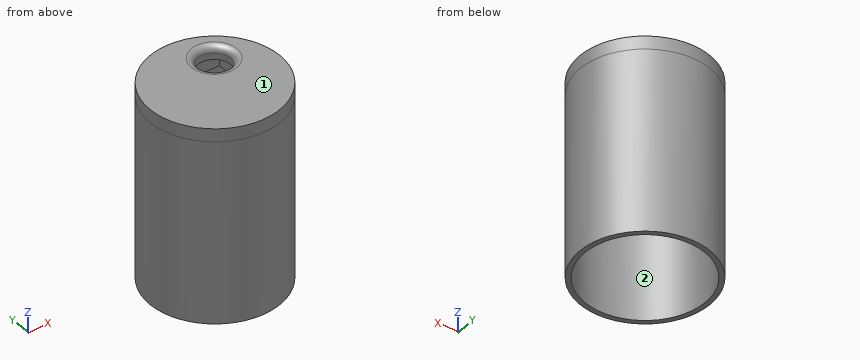
```python
from build123d import *

# Parameters (mm, degrees)
SKETCH_R      = 10
SKETCH_R_2    = 9.25
PAD_DEPTH     = 28
SKETCH001_R   = 10
SKETCH001_W   = 10.7
SKETCH001_H   = 13.5
PAD001_DEPTH  = 2
SKETCH005_R   = 10
SKETCH005_R_2 = 2.5
PAD004_DEPTH  = 2
FILLET_R      = 1


with BuildPart() as part:
    # Sketch (on XY_Plane of Origin) → Pad (new body)
    with BuildSketch(Plane.XY):
        with Locations((12, 10.7)):
            Circle(SKETCH_R)
        with Locations((12, 10.7)):
            Circle(SKETCH_R_2, mode=Mode.SUBTRACT)
    extrude(amount=-PAD_DEPTH)

    # Sketch001 (on Face3 of Pad) → Pad001 (join)
    with BuildSketch(Plane.XY):
        with Locations((12, 10.7)):
            Circle(SKETCH001_R)
        with Locations((12.5, 11.05)):
            Rectangle(SKETCH001_W, SKETCH001_H, mode=Mode.SUBTRACT)
    extrude(amount=-PAD001_DEPTH)

    # Sketch005 (on Face8 of Pad001) → Pad004 (join)
    with BuildSketch(Plane.XY):
        with Locations((12, 10.7)):
            Circle(SKETCH005_R)
        with Locations((15, 15)):
            Circle(SKETCH005_R_2, mode=Mode.SUBTRACT)
    extrude(amount=PAD004_DEPTH)

    # Fillet
    fillet_edges = [part.edges().sort_by_distance(p)[0] for p in [
        (12.5, 15, 2),
    ]]
    fillet(fillet_edges, radius=FILLET_R)


solid = part.part
```
Source: CAD feature listing. Evaluate the final solid. Frame: model axes, mm. Face numbers are marked on the shaded views. Round coordinates to 2 decimals unless told otherwise and drop trailing zeros. Order: outer loops, then holes, each group sorted by start corner. A loop starts at its lowest first (then second) coordinate and runs counter-clockwise, first axis right, second up. Notation, with made-up numbers: (14.5, -3) -> (65.5, -3) arc R19 cw to (65.5, 26) -> close; hole circle Ø8 at (4, -19.75). An arc over 180 degrees is marked (long way). Use CSV: the item, a comma, the result in double quotes.
(1) First-contact query: pin 1 Ø0.6 at (x, z) = (14, -1) entering from -Y; pin 2 Ø5.5 at (x, y) = (10, 8) entering from -Z; pin 3 Ø2 at (x, z) = (14, -1) entering from +Y. Flat tips, straight axial feed; report the tip coordinate or a pass-through.
Report:
pin 1,"y = 0.85"
pin 2,"z = 0"
pin 3,"y = 20.65"
(2) Pull-direction query (Y, two-part tool) for the marked faces 1 and 2; classes: +Y half, -Y half, draft (parallel to the pull), parting line (faces both ways), or undercut.
Report:
face 1,"draft"
face 2,"undercut"
(3) Ray query, L1, parallel to X at y = 10.5, z = -9; L2, parallel to Y at x = 12, z = -16; L3, parallel to Z at x = 18.5, y = 4.5. Return the intervals inside material, ascending.
Report:
L1,"2 to 2.75, 21.25 to 22"
L2,"0.7 to 1.45, 19.95 to 20.7"
L3,"-2 to 2"
(4) Section B-B on y = 15. Return the cut outline in (x, z), and give its area (3 significant figures).
Report:
outline,"(2.97, -28) -> (3.81, -28) -> (3.81, -2) -> (7.15, -2) -> (7.15, 0) -> (12.5, 0) -> (12.5, 1) arc R1 ccw to (11.5, 2) -> (2.97, 2) -> close; (17.5, 0) -> (17.85, 0) -> (17.85, -2) -> (20.19, -2) -> (20.19, -28) -> (21.03, -28) -> (21.03, 2) -> (18.5, 2) arc R1 ccw to (17.5, 1) -> close"
area,"84.0 mm^2"
(5) Section D-D on y = 10.7. Return the cut outline in (x, z), and give its area (3 significant figures).
Report:
outline,"(2, -28) -> (2.75, -28) -> (2.75, -2) -> (7.15, -2) -> (7.15, 0) -> (17.85, 0) -> (17.85, -2) -> (21.25, -2) -> (21.25, -28) -> (22, -28) -> (22, 2) -> (2, 2) -> close"
area,"97.6 mm^2"
(6) Section C-C on z = -9.5. Return the cut outline in (x, y), and give its area (3 significant figures).
Report:
outline,"circle Ø20 at (12, 10.7); hole circle Ø18.5 at (12, 10.7)"
area,"45.4 mm^2"
(7) Section A-A on x = 15. Return the cut outline in (y, z).
Report:
outline,"(1.16, -28) -> (1.95, -28) -> (1.95, -2) -> (4.3, -2) -> (4.3, 0) -> (12.5, 0) -> (12.5, 1) arc R1 ccw to (11.5, 2) -> (1.16, 2) -> close; (17.5, 0) -> (17.8, 0) -> (17.8, -2) -> (19.45, -2) -> (19.45, -28) -> (20.24, -28) -> (20.24, 2) -> (18.5, 2) arc R1 ccw to (17.5, 1) -> close"
